Model file for the job. Use its own axes, mm. Face numbers are marked on the shaded views. A direction names the side the tool comes from. Give positions to 0.01 mm unless a question says otherwise; leave off trailing zeros. Write each loop counter-clockwise with the first axis right and the second up, starting at its lowest first coordinate (ties: lowest second). Pieces come first, ordered by that corner, then holes. Notation, with made-up numbers: (85, -18.5) - (137, -18.5) arc R22 cw to (137, -1.5) - close; hole circle Ø8 at (-32, 41.5). An arc over 180 degrees is marked (long way). One line per item, written item: value. Start each with the question number.
(1) Cut at D-D, the plane z = 20.5. List the corners of the cut face in (x, y).
(2) Cut at A-A, the plane x = 15. List the corners of the cut face in (y, z), and give its area (3 significant figures).
(3) Drop flat-ended pins along their axis: P1, Ø1.5, axis at x = 8, y = 19, coming from the +Z side; P2, Ø10, axis at y = 27, z = 21, coming from the +X side. Give the stop position or say it passes through.
(4) Cut at C-C, the plane y = 29. List the corners of the cut face in (x, z).
(5) Probe L1, parallel to X at y = 14.5, z = 7.75; L2, parallel to Y at x = 6, z = 21.75. List the from-to ranges inside material, lowest first.
(6) 3-axis set-ups, long thin cutter, end or side, ignore diameter. For the marked faces 1 and 2: which of +Z, -Z, +X, -X, +Y, -Y reach the whole face in a straight line?
(7) Mould opens along X. For the marked faces 3, 4, 5 and 6 say: pulls with the +X half, pulls with the -X half, needs draft (parallel to the pull), parting line crosses it, or undercut.
(8) Cut at B-B, the plane y = 23. List the corners of the cut face in (x, z).
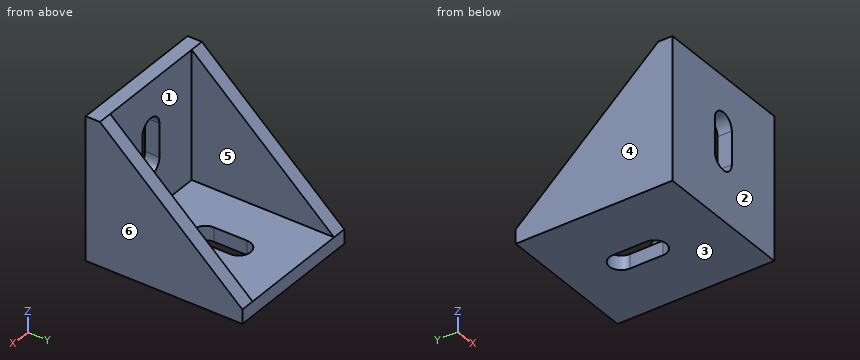
from build123d import *

# Parameters (mm, degrees)
SKETCH1_W           = 30
SKETCH1_H           = 30
BOSS_EXTRUDE1_DEPTH = 3
SKETCH2_W           = 30
SKETCH2_H           = 30
BOSS_EXTRUDE2_DEPTH = 3
BOSS_EXTRUDE3_DEPTH = 3
BOSS_EXTRUDE4_DEPTH = 3
CUT_EXTRUDE1_DEPTH  = 3
CUT_EXTRUDE2_DEPTH  = 3


with BuildPart() as part:
    # Sketch1 → Boss-Extrude1 (new body)
    with BuildSketch(Plane(origin=(0, 0, 0), x_dir=(1, 0, 0), z_dir=(0, 1, 0))):
        with Locations((15, -15)):
            Rectangle(SKETCH1_W, SKETCH1_H)
    extrude(amount=BOSS_EXTRUDE1_DEPTH)

    # Sketch2 → Boss-Extrude2 (add)
    with BuildSketch(Plane(origin=(0, 0, 0), x_dir=(-1, 0, 0), z_dir=(0, 0, -1))):
        with Locations((-15, 18)):
            Rectangle(SKETCH2_W, SKETCH2_H)
    extrude(amount=-BOSS_EXTRUDE2_DEPTH)

    # Sketch3 → Boss-Extrude3 (add)
    with BuildSketch(Plane.ZY):
        Polygon((3, 33), (3, 3), (30, 3), align=None)
    extrude(amount=-BOSS_EXTRUDE3_DEPTH)

    # Sketch4 → Boss-Extrude4 (add)
    with BuildSketch(Plane(origin=(30, 0, 0), x_dir=(0, 0, -1), z_dir=(1, 0, 0))):
        Polygon((-30, 3), (-3, 3), (-3, 33), align=None)
    extrude(amount=-BOSS_EXTRUDE4_DEPTH)

    # Sketch5 → Cut-Extrude1 (cut)
    with BuildSketch(Plane.XY.offset(3)):
        with BuildLine():
            Line((12.5, 14.5), (12.5, 21.5))
            ThreePointArc((12.5, 21.5), (15, 24), (17.5, 21.5))
            Line((17.5, 21.5), (17.5, 14.5))
            ThreePointArc((17.5, 14.5), (15, 12), (12.5, 14.5))
        make_face()
    extrude(amount=-CUT_EXTRUDE1_DEPTH, mode=Mode.SUBTRACT)

    # Sketch6 → Cut-Extrude2 (cut)
    with BuildSketch(Plane(origin=(0, 3, 0), x_dir=(1, 0, 0), z_dir=(0, 1, 0))):
        with BuildLine():
            Line((12.5, -20), (12.5, -13))
            ThreePointArc((12.5, -13), (15, -10.5), (17.5, -13))
            Line((17.5, -13), (17.5, -20))
            ThreePointArc((17.5, -20), (15, -22.5), (12.5, -20))
        make_face()
    extrude(amount=-CUT_EXTRUDE2_DEPTH, mode=Mode.SUBTRACT)


solid = part.part
Answers follow:
1. outline: (0, 0) - (12.55, 0) - (12.55, 3) - (3, 3) - (3, 13.56) - (0, 13.56) - close; (17.45, 0) - (30, 0) - (30, 13.56) - (27, 13.56) - (27, 3) - (17.45, 3) - close
2. outline: (0, 0) - (12, 0) - (12, 3) - (3, 3) - (3, 10.5) - (0, 10.5) - close; (0, 22.5) - (3, 22.5) - (3, 30) - (0, 30) - close; (24, 0) - (33, 0) - (33, 3) - (24, 3) - close
2. area: 108 mm²
3. P1: stops at z = 3
3. P2: passes through
4. outline: (0, 0) - (30, 0) - (30, 6.6) - (27, 6.6) - (27, 3) - (3, 3) - (3, 6.6) - (0, 6.6) - close
5. L1: x = 0 to 3, 27 to 30
5. L2: y = 0 to 3
6. face 1: +Z, +Y
6. face 2: +Z, -Z, +X, -X, -Y
7. face 3: needs draft
7. face 4: pulls with the -X half
7. face 5: undercut
7. face 6: pulls with the +X half
8. outline: (0, 0) - (13, 0) - (13, 3) - (3, 3) - (3, 12) - (0, 12) - close; (17, 0) - (30, 0) - (30, 12) - (27, 12) - (27, 3) - (17, 3) - close
